For this review, take the finished solid that the model builds, in its own axes (mm). Face numbers are marked on the shaded views. A direction names the side the tool comes from. Round coordinates to 2 decimals unless told otherwise and drop trailing zeros. Loops run counter-clockwise (first coordinate to the right, second up) from the corner with the lowest first, then second, coordinate; pieces in that order, holes last.
1. Clearance check with flat-ended pins moving along their axes: pin 1 Ø12.5 at (x, z) = (4.5, 24.5) entering from -Y; pin 2 Ø10 at (x, z) = (-2, 13.5) entering from +Y; pin 3 Ø12.5 at (x, z) = (3, 29.5) entering from +Y. State where each tip first meets the part, or that it passes through.
2. Consider section B-B on z = -1.5. State the section outline as (x, y) points, then the cut area to 3 significant figures.
3. To check wall thickness, follow line 1 along Z through (x, y) = (-9, 741); line 2 along Y through (x, z) = (-5, 34.5); line 3 along Y through (x, z) = (19, -2.5). State the ranges of each line that lie inside material, in increasing order.
4. Consider section A-A on x = 0. State the section outline as (y, z) points.
5. Tool access review of the marked faces 1 and 2: name each direction out of +Z, -Z, +X, -X, +Y, -Y from which nothing blocks a thin tool from reaching the whole face with its end or side.
from build123d import *

# Parameters (mm, degrees)
F0_W      = 45
F0_H      = 25
F1_DEPTH  = 800
F3_DEPTH  = 45
F5_DEPTH  = 45
F6_W      = 45
F6_H      = 25
F7_DEPTH  = 800
F9_DEPTH  = 45
F11_DEPTH = 45


with BuildPart() as f1:
    # F0 (on Front) → F1 (new body)
    with BuildSketch(Plane.XZ):
        Rectangle(F0_W, F0_H)
    extrude(amount=-F1_DEPTH)

    # F2 (on face) → F3 (cut)
    with BuildSketch(Plane.YZ.offset(22.5)):
        Polygon((0, 12.5), (0, -12.5), (25, 12.5), align=None)
    extrude(amount=-F3_DEPTH, mode=Mode.SUBTRACT)

    # F4 (on face) → F5 (cut)
    with BuildSketch(Plane(origin=(-22.5, 0, 0), x_dir=(0, -1, 0), z_dir=(-1, 0, 0))):
        Polygon((-800, 12.5), (-800, -12.5), (-775, 12.5), align=None)
    extrude(amount=-F5_DEPTH, mode=Mode.SUBTRACT)

    # F6 (on Front) → F7 (join)
    with BuildSketch(Plane.XZ):
        with Locations((0, 25)):
            Rectangle(F6_W, F6_H)
    extrude(amount=-F7_DEPTH)

    # F8 (on face) → F9 (cut)
    with BuildSketch(Plane(origin=(-22.5, 0, 0), x_dir=(0, -1, 0), z_dir=(-1, 0, 0))):
        Polygon((-730, 37.5), (-800, 37.5), (-800, 12.5), (-775, 12.5), (-730, 12.5), align=None)
    extrude(amount=-F9_DEPTH, mode=Mode.SUBTRACT)

    # F10 (on face) → F11 (cut)
    with BuildSketch(Plane(origin=(-22.5, 0, 0), x_dir=(0, -1, 0), z_dir=(-1, 0, 0))):
        Polygon((0, 12.5), (0, 37.5), (-70, 37.5), (-70, 12.5), (-25, 12.5), align=None)
    extrude(amount=-F11_DEPTH, mode=Mode.SUBTRACT)


solid = f1.part
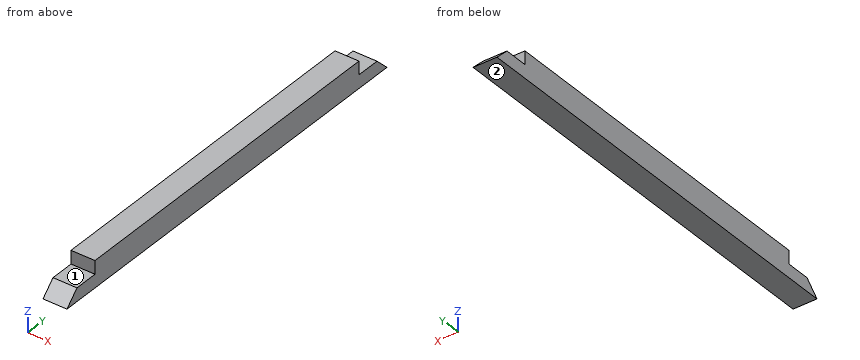
Resolved:
1. pin 1: stops at y = 70
1. pin 2: stops at y = 779
1. pin 3: stops at y = 730
2. outline: (-22.5, 11) - (22.5, 11) - (22.5, 789) - (-22.5, 789) - close
2. area: 35,000 mm2
3. line 1: z = -12.5 to 12.5
3. line 2: y = 70 to 730
3. line 3: y = 10 to 790
4. outline: (0, -12.5) - (800, -12.5) - (775, 12.5) - (730, 12.5) - (730, 37.5) - (70, 37.5) - (70, 12.5) - (25, 12.5) - close
5. face 1: +Z, +X, -X, -Y
5. face 2: -Z, +X, -X, +Y, -Y
